Geometry check sheet. Reference: drawing and pictorial views, mm from the part's lowest x, y, z. A direction names the side the tool comes from. Give positions to 0.01 mm unless a question says otherwise; leave off trailing zeros. Order: outer loops, then holes, each group sorted by start corner. A loop starts at its lowest first (then second) coordinate and runs counter-clockwise, first axis right, second up.
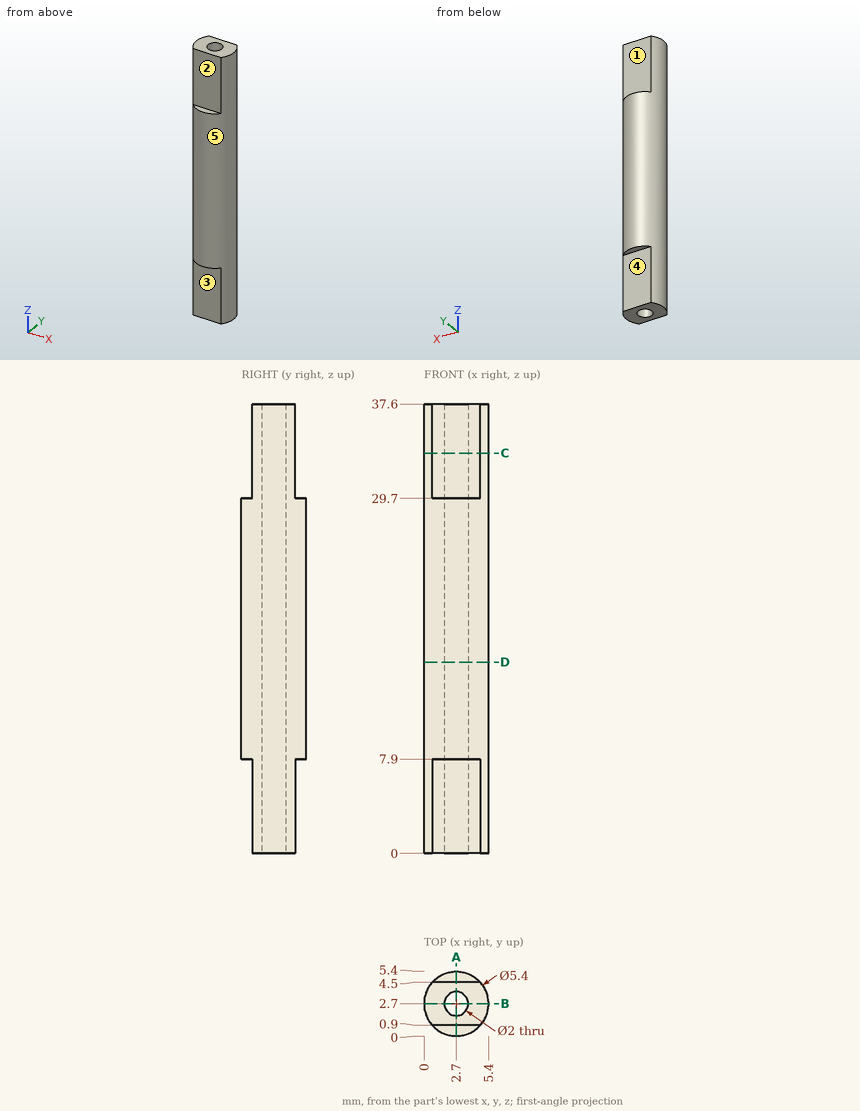
(1) Gauge pin test, flat ends, axial feed: pin 1 Ø0.7 at (x, y) = (3, 0.5) entering from +Z; pin 2 Ø0.7 at (x, y) = (3.5, 0.5) entering from -Z; pin 3 Ø1.2 at (x, z) = (3, 35.5) entering from -Y. Record the tip position at first contact, or that the pin passes through.
Response values:
pin 1: stops at z = 29.7
pin 2: stops at z = 7.9
pin 3: stops at y = 0.9
(2) Cross-section at A-A on x = 2.7. Enter the section's corners in (y, z), then the cut area to 3 significant figures.
Response values:
outline: (0, 7.9) - (0.9, 7.9) - (0.9, 0) - (1.7, 0) - (1.7, 37.6) - (0.9, 37.6) - (0.9, 29.7) - (0, 29.7) - close; (3.7, 0) - (4.5, 0) - (4.5, 7.9) - (5.4, 7.9) - (5.4, 29.7) - (4.5, 29.7) - (4.5, 37.6) - (3.7, 37.6) - close
area: 99.4 mm2
(3) Cross-section at C-C on z = 33.5. Enter the section's corners in (x, y), then the cut area to 3 significant figures.
Response values:
outline: (0.69, 0.9) - (4.71, 0.9) arc R2.7 ccw to (4.71, 4.5) - (0.69, 4.5) arc R2.7 ccw to start; hole circle Ø2 at (2.7, 2.7)
area: 14.7 mm2
(4) Cross-section at B-B on y = 2.7. Enter the section's corners in (x, z).
Response values:
outline: (0, 0) - (1.7, 0) - (1.7, 37.6) - (0, 37.6) - close; (3.7, 0) - (5.4, 0) - (5.4, 37.6) - (3.7, 37.6) - close
(5) Set-up check for the marked faces 1, 2, 3, 4 and 5: record each of +Z, -Z, +X, -X, +Y, -Y from which the full face is reachable in a straight line by a thin tool's end or side.
Response values:
face 1: +Z, +X, -X, +Y
face 2: +Z, +X, -X, -Y
face 3: -Z, +X, -X, -Y
face 4: -Z, +X, -X, +Y
face 5: +Z, -Z
(6) Cross-section at D-D on z = 16. Enter the section's corners in (x, y).
Response values:
outline: circle Ø5.4 at (2.7, 2.7); hole circle Ø2 at (2.7, 2.7)
(7) Material ranges on L1, parallel to Y at x = 2.7, z = 13; L2, parallel to Y at x = 2.65, z = 32.5; L3, parallel to Y at x = 4.55, z = 31.5, recorded low to high.
Response values:
L1: y = 0 to 1.7, 3.7 to 5.4
L2: y = 0.9 to 1.7, 3.7 to 4.5
L3: y = 0.9 to 4.5
